```python
from build123d import *

# Parameters (mm, degrees)
PAD_DEPTH                     = 28
POCKET_DEPTH                  = 22.001
SKETCH004_R                   = 1.5
PAD001_DEPTH                  = 5
SKETCH004_MIRRORED_2_R        = 1.5
PAD001_MIRRORED_2_DEPTH       = 5
SKETCH005_R                   = 1.5
POCKET001_DEPTH               = 5
SKETCH005_MIRRORED002_2_R     = 1.5
POCKET001_MIRRORED002_2_DEPTH = 5


with BuildPart() as part:
    # Sketch001 → Pad (new body)
    with BuildSketch(Plane.XY.offset(-6)):
        with BuildLine():
            Line((-48.5, 53.5), (48.5, 53.5))
            ThreePointArc((50.5, 51.5), (49.914214, 52.914214), (48.5, 53.5))
            Line((50.5, 51.5), (50.5, -51.5))
            ThreePointArc((48.5, -53.5), (49.914214, -52.914214), (50.5, -51.5))
            Line((48.5, -53.5), (-48.5, -53.5))
            ThreePointArc((-50.5, -51.5), (-49.914214, -52.914214), (-48.5, -53.5))
            Line((-50.5, -51.5), (-50.5, 51.5))
            ThreePointArc((-48.5, 53.5), (-49.914214, 52.914214), (-50.5, 51.5))
        make_face()
    extrude(amount=PAD_DEPTH)

    # Sketch002 → Pocket (cut, through all)
    with BuildSketch(Plane.XY):
        with BuildLine():
            Line((42.5, 47.5), (-42.5, 47.5))
            ThreePointArc((-42.5, 47.5), (-43.914214, 46.914214), (-44.5, 45.5))
            Line((-44.5, 45.5), (-44.5, -45.5))
            ThreePointArc((-44.5, -45.5), (-43.914214, -46.914214), (-42.5, -47.5))
            Line((-42.5, -47.5), (42.5, -47.5))
            ThreePointArc((42.5, -47.5), (43.914214, -46.914214), (44.5, -45.5))
            Line((44.5, -45.5), (44.5, 45.5))
            ThreePointArc((44.5, 45.5), (43.914214, 46.914214), (42.5, 47.5))
        make_face()
    extrude(amount=POCKET_DEPTH, mode=Mode.SUBTRACT)

    # Sketch004 → Pad001 (join)
    with BuildSketch(Plane.XY):
        with BuildLine():
            Line((-44.5, 47.5), (-29.5, 47.5))
            ThreePointArc((-44.5, 32.5), (-33.893398, 36.893398), (-29.5, 47.5))
            Line((-44.5, 47.5), (-44.5, 32.5))
        make_face()
        with Locations((-38.5, 41.5)):
            Circle(SKETCH004_R, mode=Mode.SUBTRACT)
    pad001 = extrude(amount=PAD001_DEPTH)

    # Sketch004 Mirrored 2 → Pad001 Mirrored 2 (add)
    with BuildSketch(Plane(origin=(0, 0, 0), x_dir=(-1, 0, 0), z_dir=(0, 0, -1))):
        with BuildLine():
            Line((-44.5, 47.5), (-29.5, 47.5))
            ThreePointArc((-44.5, 32.5), (-33.893398, 36.893398), (-29.5, 47.5))
            Line((-44.5, 47.5), (-44.5, 32.5))
        make_face()
        with Locations((-38.5, 41.5)):
            Circle(SKETCH004_MIRRORED_2_R, mode=Mode.SUBTRACT)
    pad001_mirrored_2 = extrude(amount=-PAD001_MIRRORED_2_DEPTH)

    # Mirrored001: Pad001, Pad001 Mirrored 2 across Sketch004 H_Axis
    add(pad001.mirror(Plane.ZX))
    add(pad001_mirrored_2.mirror(Plane.ZX))

    # Sketch005 → Pocket001 (cut)
    with BuildSketch(Plane.XY.offset(22)):
        with Locations((-46.5, 49.5)):
            Circle(SKETCH005_R)
    pocket001 = extrude(amount=-POCKET001_DEPTH, mode=Mode.SUBTRACT)

    # Sketch005 Mirrored002 2 → Pocket001 Mirrored002 2 (cut)
    with BuildSketch(Plane(origin=(0, 0, 22), x_dir=(-1, 0, 0), z_dir=(0, 0, -1))):
        with Locations((-46.5, 49.5)):
            Circle(SKETCH005_MIRRORED002_2_R)
    pocket001_mirrored002_2 = extrude(amount=POCKET001_MIRRORED002_2_DEPTH, mode=Mode.SUBTRACT)

    # Mirrored003: Pocket001, Pocket001 Mirrored002 2 across Sketch005 H_Axis
    add(pocket001.mirror(Plane(origin=(0, 0, 22), x_dir=(0, 0, 1), z_dir=(0, 1, 0))), mode=Mode.SUBTRACT)
    add(pocket001_mirrored002_2.mirror(Plane(origin=(0, 0, 22), x_dir=(0, 0, 1), z_dir=(0, 1, 0))), mode=Mode.SUBTRACT)


solid = part.part
```
Can you work these out from the model? Positions are in its coordinate system, mm. Round coordinates to 2 decimals unless told otherwise and drop trailing zeros. Order: outer loops, then holes, each group sorted by start corner. A loop starts at its lowest first (then second) coordinate and runs counter-clockwise, first axis right, second up. Notation, with made-up numbers: (18.25, 65.25) -> (54.25, 65.25) arc R9 cw to (54.25, 70.25) -> close; hole circle Ø5 at (9.5, -17.5). An arc over 180 degrees is marked (long way). Return JSON: item names as keys, results as strings. Group by question number.
1. I need wall thicknesses on line 1 (X direction, y = -49.5, z = 19.3); line 2 (Y direction, x = -46.5, z = 20.2); line 3 (X direction, y = 31, z = 14.25). Which ranges of each line are inside material? Lowest first, please. Write a range as [from, to].
2. If we section it at A-A, the plane z = 3: Write out the boundary of the cut face in (x, y), then the cut area to 3 significant figures.
3. If we section it at D-D, the plane x = -3.5: Write out the boundary of the cut face in (y, z).
4. If we section it at B-B, the plane z = 11: Write out the boundary of the cut face in (x, y).
5. Will these pins go through, and if not, where does the flat tip stop? pin 1 (1.5 mm diameter, centred on x = -46, y = 49.5, fed in from +Z); pin 2 (5 mm diameter, centred on x = 26.5, y = 14, fed in from +Z); pin 3 (3.5 mm diameter, centred on x = -38.5, y = 41.5, fed in from +Z).
6. If we section it at C-C, the plane y = 38.5: Write out the boundary of the cut face in (x, z), then the cut area to 3 significant figures.
7. We'd pull the mould along X, two halves only. Please class faces 1 (the face through (0, 48, 22)), 2 (the face through (50.5, 1, 8)), 3 (the face through (-1, 1, 0)): released by +X, released by -X, zero draft, split by the parting line, or undercut.
Output values:
{
 "1": {"line 1": "[-50.5, -48], [-45, 45], [48, 50.5]", "line 2": "[-53.5, -51], [-48, 48], [51, 53.5]", "line 3": "[-50.5, -44.5], [44.5, 50.5]"},
 "2": {"outline": "(-50.5, -51.5) arc R2 ccw to (-48.5, -53.5) -> (48.5, -53.5) arc R2 ccw to (50.5, -51.5) -> (50.5, 51.5) arc R2 ccw to (48.5, 53.5) -> (-48.5, 53.5) arc R2 ccw to (-50.5, 51.5) -> close; hole (-44.5, -32.5) arc R15 cw to (-29.5, -47.5) -> (29.5, -47.5) arc R15 cw to (44.5, -32.5) -> (44.5, 32.5) arc R15 cw to (29.5, 47.5) -> (-29.5, 47.5) arc R15 cw to (-44.5, 32.5) -> close; hole circle Ø3 at (-38.5, -41.5); hole circle Ø3 at (-38.5, 41.5); hole circle Ø3 at (38.5, -41.5); hole circle Ø3 at (38.5, 41.5)", "area": "3,030 mm²"},
 "3": {"outline": "(-53.5, -6) -> (53.5, -6) -> (53.5, 22) -> (47.5, 22) -> (47.5, 0) -> (-47.5, 0) -> (-47.5, 22) -> (-53.5, 22) -> close"},
 "4": {"outline": "(-50.5, -51.5) arc R2 ccw to (-48.5, -53.5) -> (48.5, -53.5) arc R2 ccw to (50.5, -51.5) -> (50.5, 51.5) arc R2 ccw to (48.5, 53.5) -> (-48.5, 53.5) arc R2 ccw to (-50.5, 51.5) -> close; hole (-44.5, -45.5) arc R2 ccw to (-42.5, -47.5) -> (42.5, -47.5) arc R2 ccw to (44.5, -45.5) -> (44.5, 45.5) arc R2 ccw to (42.5, 47.5) -> (-42.5, 47.5) arc R2 ccw to (-44.5, 45.5) -> close"},
 "5": {"pin 1": "z = 17", "pin 2": "z = 0", "pin 3": "z = 5"},
 "6": {"outline": "(-50.5, -6) -> (50.5, -6) -> (50.5, 22) -> (44.5, 22) -> (44.5, 5) -> (32.5, 5) -> (32.5, 0) -> (-32.5, 0) -> (-32.5, 5) -> (-44.5, 5) -> (-44.5, 22) -> (-50.5, 22) -> close", "area": "990 mm²"},
 "7": {"face 1": "zero draft", "face 2": "released by +X", "face 3": "undercut"}
}
